Read the model definition and answer for the solid it produces. Units are mm, in the model's axes. A direction names the side the tool comes from. Coordinates: 2 decimals unless noted, no trailing zeros. Order: outer loops, then holes, each group sorted by start corner. A loop starts at its lowest first (then second) coordinate and runs counter-clockwise, first axis right, second up. Notation, with made-up numbers: (-22.5, 76) -> (-5.5, 76) arc R20 ccw to (-5.5, 87) -> close; hole circle Ø10 at (73, 85). An arc over 180 degrees is marked (long way). Answer in a Markdown table with one row per item.
from build123d import *

# Parameters (mm, degrees)
SKETCH_1_R          = 17.45
EXTRUDE_1_DEPTH     = 3
SKETCH_2_R          = 14.95
EXTRUDE_2_DEPTH     = 27
SKETCH_4_R          = 12.5
EXTRUDE_3_DEPTH     = 22
SKETCH_5_R          = 12
EXTRUDE_4_DEPTH     = 12
CHAMFER_1_SIZE      = 0.5
SKETCH_6_W          = 1
SKETCH_6_H          = 2
CHAMFER_2_SIZE      = 0.5
CHAMFER_3_SIZE      = 1
SKETCH_7_W          = 12
SKETCH_7_H          = 5
CUT_EXTRUDE_1_DEPTH = 3
FILLET_1_R          = 2.5


with BuildPart() as part:
    # 草图1 → 拉伸1 (new body)
    with BuildSketch(Plane.XY):
        Circle(SKETCH_1_R)
    extrude(amount=EXTRUDE_1_DEPTH)

    # 草图2 → 拉伸2 (add)
    with BuildSketch(Plane.XY.offset(3)):
        Circle(SKETCH_2_R)
    extrude(amount=EXTRUDE_2_DEPTH)

    # 草图4 → 拉伸3 (add)
    with BuildSketch(Plane.XY.offset(30)):
        Circle(SKETCH_4_R)
    extrude(amount=EXTRUDE_3_DEPTH)

    # 草图5 → 拉伸4 (add)
    with BuildSketch(Plane.XY.offset(52)):
        Circle(SKETCH_5_R)
    extrude(amount=EXTRUDE_4_DEPTH)

    # 倒角1
    chamfer_1_edges = [part.edges().sort_by_distance(p)[0] for p in [
        (-12, 0, 64),
    ]]
    chamfer(chamfer_1_edges, length=CHAMFER_1_SIZE)

    # 草图6 → 切除-旋转1 (revolve, cut)
    with BuildSketch(Plane(origin=(0, 0, 0), x_dir=(1, 0, 0), z_dir=(0, 1, 0)), mode=Mode.PRIVATE) as cut_revolve_1_sk:
        with Locations((-11.5, -53)):
            Rectangle(SKETCH_6_W, SKETCH_6_H)
    revolve(cut_revolve_1_sk.sketch.rotate(Axis((0, 0, 52), (0, 0, -1)), 180), axis=Axis((0, 0, 52), (0, 0, -1)), mode=Mode.SUBTRACT)

    # 倒角2
    chamfer_2_edges = [part.edges().sort_by_distance(p)[0] for p in [
        (-12.5, 0, 52),
        (-17.45, 0, 3),
        (-14.95, 0, 30),
    ]]
    chamfer(chamfer_2_edges, length=CHAMFER_2_SIZE)

    # 倒角3
    chamfer_3_edges = [part.edges().sort_by_distance(p)[0] for p in [
        (-17.45, 0, 0),
    ]]
    chamfer(chamfer_3_edges, length=CHAMFER_3_SIZE)

    # 草图7 → 切除-拉伸1 (cut)
    with BuildSketch(Plane(origin=(12, 0, 0), x_dir=(0, 0, -1), z_dir=(1, 0, 0))):
        with Locations((-58, 0)):
            Rectangle(SKETCH_7_W, SKETCH_7_H)
    extrude(amount=-CUT_EXTRUDE_1_DEPTH, mode=Mode.SUBTRACT)

    # 圆角1
    # the kernel refuses this fillet: 2.5 mm, written as the material it adds along each edge
    with BuildSketch(Plane(origin=(16.962142643, -2.5, 52), x_dir=(0, 1, 0), z_dir=(-1, 0, 0))) as fillet_1_piece_1_section:
        with BuildLine():
            CenterArc((FILLET_1_R, -FILLET_1_R), FILLET_1_R, 90, 90)
            Line((0, -FILLET_1_R), (0, 0))
            Line((0, 0), (FILLET_1_R, 0))
        make_face()
    fillet_1_piece_1 = extrude(amount=14.212142643, mode=Mode.PRIVATE)
    fillet_1_piece_1 = fillet_1_piece_1 & Plane(origin=(0, 0, 54.124758418), x_dir=(1, 0, 0), z_dir=(0, 0, -1)) * Cylinder(12, 39, mode=Mode.PRIVATE)
    fillet_1_piece_1 = split(fillet_1_piece_1, bisect_by=Plane(origin=(11.227777132, -2.484876178, 54), z_dir=(0, 0, 1)), keep=Keep.TOP, mode=Mode.PRIVATE)
    add(fillet_1_piece_1)
    with BuildSketch(Plane(origin=(16.962142643, -2.5, 52), x_dir=(0, 1, 0), z_dir=(-1, 0, 0))) as fillet_1_piece_2_section:
        with BuildLine():
            CenterArc((FILLET_1_R, -FILLET_1_R), FILLET_1_R, 90, 90)
            Line((0, -FILLET_1_R), (0, 0))
            Line((0, 0), (FILLET_1_R, 0))
        make_face()
    fillet_1_piece_2 = extrude(amount=14.212142643, mode=Mode.PRIVATE)
    fillet_1_piece_2 = fillet_1_piece_2 & Plane(origin=(0, 0, 53.528388409), x_dir=(1, 0, 0), z_dir=(0, 0, 1)) * Cylinder(11, 39, mode=Mode.PRIVATE)
    add(fillet_1_piece_2)
    with BuildSketch(Plane(origin=(16.962142643, 2.5, 52), x_dir=(0, -1, 0), z_dir=(-1, 0, 0))) as fillet_1_piece_3_section:
        with BuildLine():
            CenterArc((FILLET_1_R, FILLET_1_R), FILLET_1_R, 180, 90)
            Line((0, FILLET_1_R), (0, 0))
            Line((0, 0), (FILLET_1_R, 0))
        make_face()
    fillet_1_piece_3 = extrude(amount=14.212142643, mode=Mode.PRIVATE)
    fillet_1_piece_3 = fillet_1_piece_3 & Plane(origin=(0, 0, 54.124758418), x_dir=(1, 0, 0), z_dir=(0, 0, -1)) * Cylinder(12, 39, mode=Mode.PRIVATE)
    fillet_1_piece_3 = split(fillet_1_piece_3, bisect_by=Plane(origin=(11.227777136, 2.484876178, 54), z_dir=(0, 0, 1)), keep=Keep.TOP, mode=Mode.PRIVATE)
    add(fillet_1_piece_3)
    with BuildSketch(Plane(origin=(16.962142643, 2.5, 52), x_dir=(0, -1, 0), z_dir=(-1, 0, 0))) as fillet_1_piece_4_section:
        with BuildLine():
            CenterArc((FILLET_1_R, FILLET_1_R), FILLET_1_R, 180, 90)
            Line((0, FILLET_1_R), (0, 0))
            Line((0, 0), (FILLET_1_R, 0))
        make_face()
    fillet_1_piece_4 = extrude(amount=14.212142643, mode=Mode.PRIVATE)
    fillet_1_piece_4 = fillet_1_piece_4 & Plane(origin=(0, 0, 53.5283884), x_dir=(1, 0, 0), z_dir=(0, 0, 1)) * Cylinder(11, 39, mode=Mode.PRIVATE)
    add(fillet_1_piece_4)


solid = part.part
Q1. The part is cut by section B-B (z = 56.5). Write down the section's boundary in (x, y).
Outcome:
| item | result |
|---|---|
| outline | (9, -2.5) -> (9, 2.5) -> (11.74, 2.5) arc R12 ccw (long way) to (11.74, -2.5) -> close |
Q2. The part is cut by section C-C (z = 15.5). Write down the section's boundary in (x, y).
Outcome:
| item | result |
|---|---|
| outline | circle Ø29.9 at (0, 0) |
Q3. Consider line 1 (Z direction, x = -15, y = 6.5); line 2 (X direction, y = -0.5, z = 26.5); line 3 (Z direction, x = 2, y = 11.5). Determine where each line is inside the solid, lowest interval first.
Outcome:
| item | result |
|---|---|
| line 1 | 0 to 3 |
| line 2 | -14.94 to 14.94 |
| line 3 | 0 to 52, 54 to 63.83 |
Q4. For faces 4 (the face through (10, -2.5, 59)), 5 (the face through (-3.783, -17.035, 1.74)), 6 (the face through (10, -5, 52)), 7 (the face through (11.923, 3.755, 40.6)), determine the directions among +Z, -Z, +X, -X, +Y, -Y from which every point of the face is accessible in a straight line to the end or side of a thin tool.
Outcome:
| item | result |
|---|---|
| face 4 | +Z, +X |
| face 5 | +Z, -Z |
| face 6 | none |
| face 7 | +Z |
Q5. For a pull along Z with two mould halves and no side action, classify faces 1 (the face through (0, 0, 64)), 2 (the face through (-11, -3, 54)), 3 (the face through (0, 0, 0)) as pulls with the +Z half, pulls with the -Z half, needs draft (parallel to the pull), parting line crosses it, or undercut.
Outcome:
| item | result |
|---|---|
| face 1 | pulls with the +Z half |
| face 2 | undercut |
| face 3 | pulls with the -Z half |
Q6. Given pin 1 (12 mm diameter, centred on x = -5.5, z = 44, fed in from -Y); pin 2 (3 mm diameter, centred on y = 8, z = 24, fed in from -X); pin 3 (2 mm diameter, centred on x = 13.5, y = 6.5, fed in from +Z), each flat-ended and moving along its own axis, determine where each tip first touches the part or whether it passes through.
Outcome:
| item | result |
|---|---|
| pin 1 | y = -12.5 |
| pin 2 | x = -13.46 |
| pin 3 | z = 30 |
